from build123d import *

# Parameters (mm, degrees)
F1_DEPTH = 25
F2_R     = 5


# Not quite as in the source:
# - the program builds the solid bodies; features that only make, move or delete a surface that nothing else refers to are left out


with BuildPart() as f1:
    # F0 (on Front) → F1 (new body)
    with BuildSketch(Plane.XZ):
        with BuildLine():
            ThreePointArc((22.5237740783, 50.7157030305), (18.9120996382, 45.5821277938), (12.9524584639, 43.6122384452))
            Line((12.9524584639, 43.6122384452), (-35.9964722395, 43.6122384452))
            ThreePointArc((-35.9964722395, 43.6122384452), (-43.0675400514, 40.6833062571), (-45.9964722395, 33.6122384452))
            Line((-45.9964722395, 33.6122384452), (-45.9964722395, -33.6122384452))
            ThreePointArc((-45.9964722395, -33.6122384452), (-43.0675400514, -40.6833062571), (-35.9964722395, -43.6122384452))
            Line((-35.9964722395, -43.6122384452), (35.9964722395, -43.6122384452))
            ThreePointArc((35.9964722395, -43.6122384452), (43.0675400514, -40.6833062571), (45.9964722395, -33.6122384452))
            Line((45.9964722395, -33.6122384452), (45.9964722395, 10.5682246696))
            ThreePointArc((45.9964722395, 10.5682246696), (47.9663615881, 16.5278658439), (53.0999368248, 20.139540284))
            ThreePointArc((53.0999368248, 20.139540284), (63.3375617105, 60.9533279162), (22.5237740783, 50.7157030305))
        make_face()
    extrude(amount=F1_DEPTH)

    # F2
    f2_edges = [f1.edges().sort_by_distance(p)[0] for p in [
        (63.337562, -25, 60.953328),
        (63.337562, 0, 60.953328),
    ]]
    fillet(f2_edges, radius=F2_R)


solid = f1.part
Here's how the part is built. I have some questions about the finished solid (model axes, mm). A direction names the side the tool comes from. Give positions to 0.01 mm unless a question says otherwise; leave off trailing zeros. Write each loop counter-clockwise with the first axis right and the second up, starting at its lowest first coordinate (ties: lowest second). Pieces come first, ordered by that corner, then holes. Notation, with made-up numbers: (53.5, 42) -> (102.5, 42) arc R14 ccw to (102.5, 68) -> close; hole circle Ø6 at (46.25, 26). An arc over 180 degrees is marked (long way). Use one line per item in the form item = value. Start each with the question number.
1. If I drill on L1, parallel to Z at x = -35, y = -12; L2, parallel to X at y = -5, z = 62; L3, parallel to X at y = -13, z = 33, over which ranges is the centre line in solid material (lowest first)?
2. Imagine slicing it at C-C on z = -11. List the corners of the cut face in (x, y) for me.
3. Imagine slicing it at B-B on y = -18.25. List the corners of the cut face in (x, z) for me, plus the area to 3 significant figures.
4. On a 3-axis mill with a long thin cutter (end or side, diameter ignored), from which of +Z, -Z, +X, -X, +Y, -Y can I reach the whole of each face in a straight line? I mean faces 1 (the face through (-11.865, -1.504, 42.186)), 2 (the face through (44.571, -1.504, -11.213)), 3 (the face through (45.996, -12, -12)), 4 (the face through (-11.865, -23.496, 42.186)). Say none if no direction works.
5. Will these pins go through, and if not, where does the flat tip stop? pin 1 Ø12 at (x, y) = (37.5, -8) entering from -Z; pin 2 Ø4.5 at (y, z) = (-10, -2.5) entering from +X; pin 3 Ø6 at (x, y) = (-31, -20) entering from +Z; pin 4 Ø6 at (y, z) = (-14, 38.5) entering from -X.
6. Imagine slicing it at A-A on x = -18. List the corners of the cut face in (y, z) for me.
Entries:
q1.L1 = -43.61 to 43.61
q1.L2 = 29.77 to 62.22
q1.L3 = -46 to 68.11
q2.outline = (-46, -20) arc R5 ccw to (-41, -25) -> (41, -25) arc R5 ccw to (46, -20) -> (46, -5) arc R5 ccw to (41, 0) -> (-41, 0) arc R5 ccw to (-46, -5) -> close
q3.outline = (-46, -33.61) arc R10 ccw to (-36, -43.61) -> (36, -43.61) arc R10 ccw to (46, -33.61) -> (46, 10.57) arc R10 cw to (53.1, 20.14) arc R24.52 ccw (long way) to (22.52, 50.72) arc R10 cw to (12.95, 43.61) -> (-36, 43.61) arc R10 ccw to (-46, 33.61) -> close
q3.area = 9,400 mm²
q4.face_1 = +Z, -X, +Y
q4.face_2 = -Z, +X, +Y
q4.face_3 = -Z, +X, +Y, -Y
q4.face_4 = +Z, -X, -Y
q5.pin_1 = -43.61
q5.pin_2 = 46
q5.pin_3 = 43.61
q5.pin_4 = -45.82
q6.outline = (-25, -38.61) arc R5 ccw to (-20, -43.61) -> (-5, -43.61) arc R5 ccw to (0, -38.61) -> (0, 38.61) arc R5 ccw to (-5, 43.61) -> (-20, 43.61) arc R5 ccw to (-25, 38.61) -> close
